Build history of the part. All positions in model axes, mm. A direction names the side the tool comes from. Round coordinates to 2 decimals unless told otherwise and drop trailing zeros. Order: outer loops, then holes, each group sorted by start corner. A loop starts at its lowest first (then second) coordinate and runs counter-clockwise, first axis right, second up. Notation, with made-up numbers: M 8,1.25 L 62,1.25 A11 ccw 62,19.25 Z; hole C 13.25,-14 d2. An arc over 180 degrees is marked long. One line per item, written item: value. Start each with the question number.
Item 1: Band-saw the part on C-C, the plane y = 0. Write the cut outline in (x, z).
Item 2: Tool access for faces 1 (the flat face through (197.91, 17, -17)), 2 (the flat face through (-50, 14, 21)), 3 (the cylindrical face through (126, -22.2, -11.5)): list every direction of +Z, -Z, +X, -X, +Y, -Y with a clear straight run to the whole face (end or side of a thin tool).
Item 3: Probe L1, parallel to Z at x = 114, y = 0.5 (3 decimals); L2, parallel to X at y = 27, z = 6.5; L3, parallel to X at y = 20, z = -14. List the from-to ranges inside material, lowest first.
Item 4: Two-plate mould, pull along X, no slides. Class faces 4 (the flat face through (207.91, 0, 0)), 5 (the flat face through (-200, 0, 0)), 6 (the cylindrical face through (0.7, 30.736, 4.036)), 7 (the cylindrical face through (199.6, 7.1, -22.4)): +X half, -X half, draft (parallel to the pull), parting line (faces both ways), or undercut.
Item 5: Band-saw the part on D-D, the plane x = -112. Write the cut outline in (y, z), then the cut area to 3 significant figures.
Item 6: Band-saw the part on A-A, the plane z = 0. Write the cut outline in (x, y) (3 decimals).
Item 7: Pin check, flat tips, straight feed: pin 1 (8 mm diameter, centred on x = 50, z = -2.5, fed in from +Y); pin 2 (1 mm diameter, centred on x = 9.5, y = 18, fed in from -Z); pin 3 (3 mm diameter, centred on x = 164, y = -20.5, fed in from -Z). Stop position of each tip, or through.
Item 8: Band-saw the part on B-B, the plane x = 132.5. Write the cut outline in (y, z), then the cut area to 3 significant figures.
```python
from build123d import *

# Parameters (mm, degrees)
SKETCH1_R           = 31
SKETCH1_R_2         = 25
BOSS_EXTRUDE1_DEPTH = 50
SKETCH1_4_R         = 25
BOSS_EXTRUDE2_DEPTH = 200
CUT_EXTRUDE1_START  = 130.215
CUT_EXTRUDE1_DEPTH  = 100.215
BOSS_EXTRUDE3_START = 7.91
SKETCH5_R           = 25
BOSS_EXTRUDE3_DEPTH = 7.91
CUT_EXTRUDE2_START  = -6.6
SKETCH6_R           = 25
SKETCH6_R_2         = 23.5
CUT_EXTRUDE2_DEPTH  = 3.4


with BuildPart() as part:
    # Sketch1 → Boss-Extrude1 (new, symmetric)
    # profile 1 of 2: a face of its own
    with BuildSketch(Plane(origin=(0, 0, 0), x_dir=(0, 0, -1), z_dir=(1, 0, 0))):
        Circle(SKETCH1_R)
        Circle(SKETCH1_R_2, mode=Mode.SUBTRACT)
    # profile 2 of 2: a face of its own
    with BuildSketch(Plane(origin=(0, 0, 0), x_dir=(0, 0, -1), z_dir=(1, 0, 0))):
        Circle(SKETCH1_R_2)
    extrude(amount=BOSS_EXTRUDE1_DEPTH, both=True)

    # Sketch1_4 → Boss-Extrude2 (add, symmetric)
    with BuildSketch(Plane(origin=(0, 0, 0), x_dir=(0, 0, -1), z_dir=(1, 0, 0))):
        Circle(SKETCH1_4_R)
    extrude(amount=BOSS_EXTRUDE2_DEPTH, both=True)

    # Sketch3 → Cut-Revolve1 (revolve, cut)
    with BuildSketch(Plane.XY, mode=Mode.PRIVATE) as cut_revolve1_sk:
        with BuildLine():
            Line((52, 25), (50, 25))
            ThreePointArc((50, 25), (51, 24), (52, 25))
        make_face()
        with BuildLine():
            Line((-52, 25), (-50, 25))
            ThreePointArc((-50, 25), (-51, 24), (-52, 25))
        make_face()
    revolve(cut_revolve1_sk.sketch.rotate(Axis((0, 0, 0), (1, 0, 0)), 90), axis=Axis((0, 0, 0), (1, 0, 0)), mode=Mode.SUBTRACT)

    # Sketch4 → Cut-Extrude1 (cut)
    with BuildSketch(Plane(origin=(50, 0, 0), x_dir=(0, 0, -1), z_dir=(1, 0, 0)).offset(CUT_EXTRUDE1_START)):
        with BuildLine():
            Line((-8, 23.685438565), (-8, 19.6))
            ThreePointArc((-8, 19.6), (-7.912132034, 19.387867966), (-7.7, 19.3))
            Line((-7.7, 19.3), (7.7, 19.3))
            ThreePointArc((7.7, 19.3), (7.912132034, 19.387867966), (8, 19.6))
            Line((8, 19.6), (8, 23.685438565))
            ThreePointArc((8, 23.685438565), (0, 25), (-8, 23.685438565))
        make_face()
    extrude(amount=-CUT_EXTRUDE1_DEPTH, mode=Mode.SUBTRACT)

    # Sketch5 → Boss-Extrude3 (add)
    with BuildSketch(Plane(origin=(200, 0, 0), x_dir=(0, 0, -1), z_dir=(1, 0, 0)).offset(BOSS_EXTRUDE3_START)):
        with Locations(Location((0, 0, 0), (0, 0, 180))):
            Circle(SKETCH5_R)
    extrude(amount=-BOSS_EXTRUDE3_DEPTH)

    # Sketch6 → Cut-Extrude2 (cut)
    with BuildSketch(Plane(origin=(207.91, 0, 0), x_dir=(0, 0, -1), z_dir=(1, 0, 0)).offset(CUT_EXTRUDE2_START)):
        with Locations(Location((0, 0, 0), (0, 0, 180))):
            Circle(SKETCH6_R)
        Circle(SKETCH6_R_2, mode=Mode.SUBTRACT)
    extrude(amount=-CUT_EXTRUDE2_DEPTH, mode=Mode.SUBTRACT)


solid = part.part
```
Output:
1. outline: M -200,-25 L -52,-25 A1 cw -50,-25 L -50,-31 L 50,-31 L 50,-25 A1 cw 52,-25 L 197.91,-25 L 197.91,-23.5 L 201.31,-23.5 L 201.31,-25 L 207.91,-25 L 207.91,25 L 201.31,25 L 201.31,23.5 L 197.91,23.5 L 197.91,25 L 52,25 A1 cw 50,25 L 50,31 L -50,31 L -50,25 A1 cw -52,25 L -200,25 Z
2. face 1: none
2. face 2: -X
2. face 3: +X
3. L1: z = -24.995 to 24.995
3. L2: x = -50 to 50
3. L3: x = -200 to -51.81, -50.19 to 50.19, 51.81 to 197.91, 201.31 to 207.91
4. face 4: +X half
4. face 5: -X half
4. face 6: draft
4. face 7: undercut
5. outline: C 0,0 d50
5. area: 1,960 mm²
6. outline: M -200,-25 L -52,-25 A1 cw -50,-25 L -50,-31 L 50,-31 L 50,-25 A1 cw 52,-25 L 197.91,-25 L 197.91,-23.5 L 201.31,-23.5 L 201.31,-25 L 207.91,-25 L 207.91,25 L 201.31,25 L 201.31,23.5 L 197.91,23.5 L 197.91,25 L 180.215,25 L 180.215,19.3 L 80,19.3 L 80,25 L 52,25 A1 cw 50,25 L 50,31 L -50,31 L -50,25 A1 cw -52,25 L -200,25 Z
7. pin 1: stops at y = 31
7. pin 2: stops at z = -25.59
7. pin 3: stops at z = -16.25
8. outline: M 19.3,-7.7 L 19.3,7.7 A0.3 cw 19.6,8 L 23.69,8 A25 ccw long 23.69,-8 L 19.6,-8 A0.3 cw Z
8. area: 1,880 mm²
